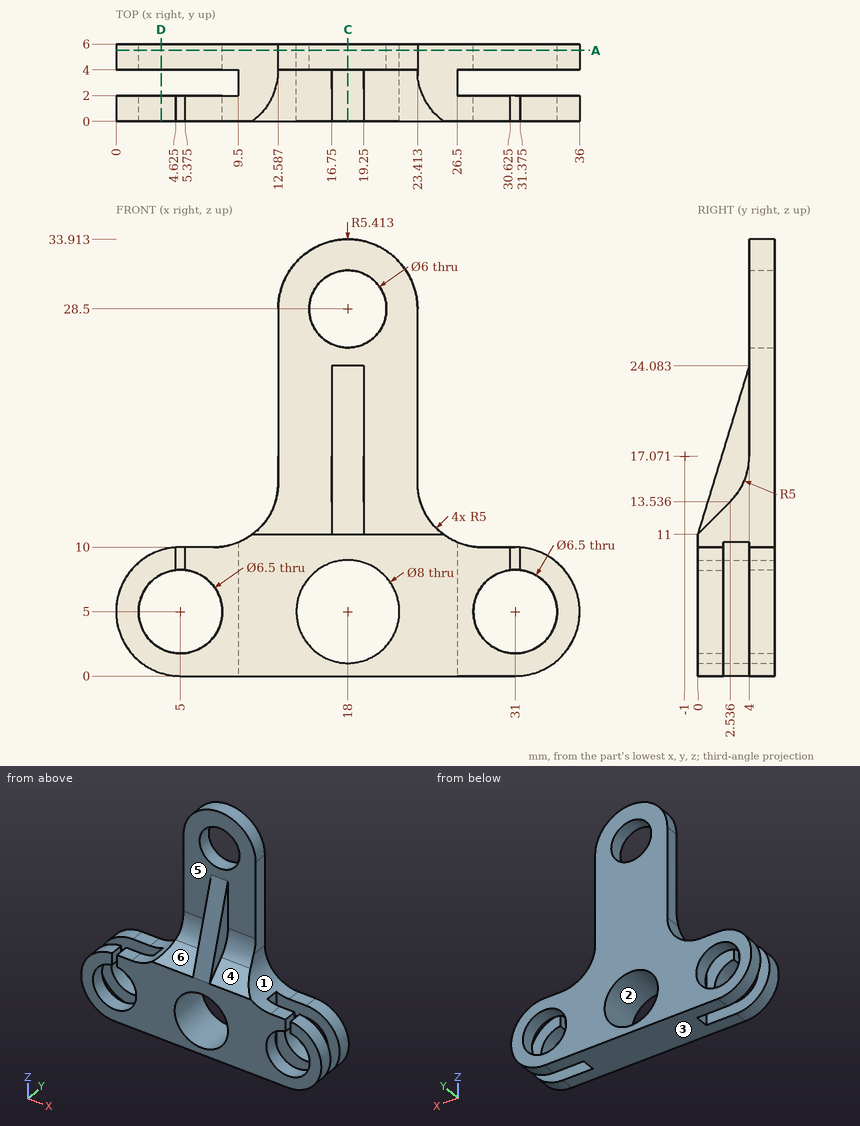
Study the drawing (mm; zero at the part's minimum x, y, z) and answer. A direction names the side the tool comes from. Round coordinates to 2 decimals unless told otherwise and drop trailing zeros. Loops run counter-clockwise (first coordinate to the right, second up) from the corner with the lowest first, then second, coordinate; pieces in that order, holes last. Notation, with made-up numbers: (18, -33) - (62, -33) arc R13 ccw to (62, -11) - close; hole circle Ø1 at (6.25, 60). An arc over 180 degrees is marked (long way). Use one line per item in the form item = value. Start each with the question number.
1. The part is cut by section A-A on y = 5.5. Give the number of separate pieces and of enclosed holes in the cut face.
2. For a pull along X with two mould halves and no side action, classify the marked faces 1, 2 and 3 as pulls with the +X half, pulls with the -X half, needs draft (parallel to the pull), parting line crosses it, or undercut.
3. Consider line 1 (Z direction, x = 16.5, y = 5.75); line 2 (X direction, y = 5.25, z = 28.5); line 3 (Z direction, x = 18, y = 5.2). Determine where each line is inside the solid, lowest interval first. Write a range as [from, to].
4. A tool of negligible diameter and unlimited length cuts with its end or side. For the marked faces 4, 5 and 6, from which of +Z, -Z, +X, -X, +Y, -Y can it reach the whole face along a straight path? Write none if from no direction.
5. The part is cut by section C-C on x = 18. Determine the outline of the cut face in (y, z).
6. The part is cut by section D-D on x = 3.5. Determine the outline of the cut face in (y, z).
7. Given pin 1 Ø1.6 at (x, y) = (6.5, 1.5) entering from +Z; pin 2 Ø10.5 at (x, z) = (31, 5) entering from -Y; pin 3 Ø3 at (y, z) = (2.5, 16.5) entering from +X; pin 4 Ø0.9 at (y, z) = (0.5, 9) entering from +X, each flat-ended and moving along its own axis, determine where each tip first touches the part or whether it passes through.
Geometry check:
q1.separate_pieces = 1
q1.enclosed_holes = 4
q2.face_1 = pulls with the +X half
q2.face_2 = undercut
q2.face_3 = needs draft
q3.line_1 = [0, 1.29], [8.71, 25.9], [31.1, 33.7]
q3.line_2 = [12.59, 15], [21, 23.41]
q3.line_3 = [0, 1], [9, 25.5], [31.5, 33.91]
q4.face_4 = +Z, +X, -Y
q4.face_5 = +Z, -Y
q4.face_6 = +Z, -X, -Y
q5.outline = (0, 0) - (6, 0) - (6, 1) - (0, 1) - close; (0, 9) - (6, 9) - (6, 25.5) - (4, 25.5) - (4, 24.08) - (0, 11) - close; (4, 31.5) - (6, 31.5) - (6, 33.91) - (4, 33.91) - close
q6.outline = (0, 0.23) - (2, 0.23) - (2, 2.12) - (0, 2.12) - close; (0, 7.88) - (2, 7.88) - (2, 9.77) - (0, 9.77) - close; (4, 0.23) - (6, 0.23) - (6, 2.12) - (4, 2.12) - close; (4, 7.88) - (6, 7.88) - (6, 9.77) - (4, 9.77) - close
q7.pin_1 = 10
q7.pin_2 = 0
q7.pin_3 = 23.41
q7.pin_4 = 34.52
